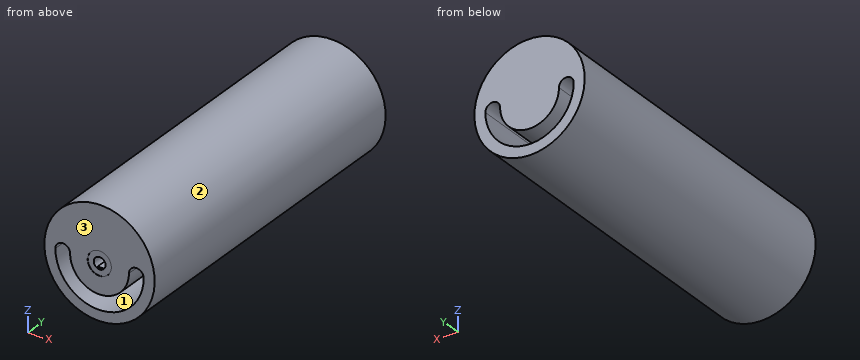
```python
from build123d import *

# Parameters (mm, degrees)
SKETCH1_R           = 28.1
BOSS_EXTRUDE2_DEPTH = 61.3
SKETCH3_R           = 18.6
CUT_EXTRUDE2_DEPTH  = 58.8
SKETCH4_W           = 56.2
SKETCH4_H           = 56.2
BOSS_EXTRUDE3_DEPTH = 56.2
SKETCH5_R           = 16.1
CUT_EXTRUDE4_DEPTH  = 5
SKETCH6_W           = 49.797391422
SKETCH6_H           = 49.779255452
CUT_EXTRUDE5_DEPTH  = 53.7
SKETCH7_R           = 28.1
BOSS_EXTRUDE4_DEPTH = 321.5
CUT_EXTRUDE6_DEPTH  = 10
SKETCH9_R           = 3
CUT_EXTRUDE7_DEPTH  = 1
SKETCH10_R          = 6.025
CUT_EXTRUDE8_DEPTH  = 0.1
SKETCH18_R          = 3.75
CUT_EXTRUDE9_DEPTH  = 100
SKETCH19_R          = 3.75
CUT_EXTRUDE11_DEPTH = 325
SKETCH20_W          = 56.2
SKETCH20_H          = 56.2
CUT_EXTRUDE13_DEPTH = 200
SKETCH21_R          = 28.1
CUT_EXTRUDE14_DEPTH = 150


with BuildPart() as part:
    # Sketch1 → Boss-Extrude2 (new body)
    with BuildSketch(Plane.XY):
        Circle(SKETCH1_R)
    extrude(amount=BOSS_EXTRUDE2_DEPTH)

    # Sketch3 → Cut-Extrude2 (cut)
    with BuildSketch(Plane.XY.offset(61.3)):
        with Locations((0, -7)):
            Circle(SKETCH3_R)
    extrude(amount=-CUT_EXTRUDE2_DEPTH, mode=Mode.SUBTRACT)

    # Sketch4 → Boss-Extrude3 (add)
    with BuildSketch(Plane(origin=(0, 0, 0), x_dir=(-1, 0, 0), z_dir=(0, 0, -1))):
        Rectangle(SKETCH4_W, SKETCH4_H)
    extrude(amount=BOSS_EXTRUDE3_DEPTH)

    # Sketch5 → Cut-Extrude4 (cut)
    with BuildSketch(Plane.XY.offset(2.5)):
        with Locations((0, -7)):
            Circle(SKETCH5_R)
    extrude(amount=-CUT_EXTRUDE4_DEPTH, mode=Mode.SUBTRACT)

    # Sketch6 → Cut-Extrude5 (cut)
    with BuildSketch(Plane(origin=(0, 0, -56.2), x_dir=(-1, 0, 0), z_dir=(0, 0, -1))):
        Rectangle(SKETCH6_W, SKETCH6_H)
    extrude(amount=-CUT_EXTRUDE5_DEPTH, mode=Mode.SUBTRACT)

    # Sketch7 → Boss-Extrude4 (add)
    with BuildSketch(Plane(origin=(0, -28.1, 0), x_dir=(-1, 0, 0), z_dir=(0, -1, 0))):
        with Locations(Location((0, 28.1, 0), (0, 0, 90))):
            Circle(SKETCH7_R)
    extrude(amount=BOSS_EXTRUDE4_DEPTH)

    # Sketch8 → Cut-Extrude6 (cut)
    with BuildSketch(Plane(origin=(0, -349.6, 0), x_dir=(-1, 0, 0), z_dir=(0, -1, 0))):
        with BuildLine():
            Line((-1.658312395, 25.832078896), (1.658312395, 25.832078896))
            ThreePointArc((1.658312395, 25.832078896), (3, 28.332078896), (1.658312395, 30.832078896))
            Line((1.658312395, 30.832078896), (-1.658312395, 30.832078896))
            ThreePointArc((-1.658312395, 30.832078896), (-3, 28.332078896), (-1.658312395, 25.832078896))
        make_face()
    extrude(amount=-CUT_EXTRUDE6_DEPTH, mode=Mode.SUBTRACT)

    # Sketch9 → Cut-Extrude7 (cut)
    with BuildSketch(Plane(origin=(0, -349.6, 0), x_dir=(-1, 0, 0), z_dir=(0, -1, 0))):
        with Locations(Location((0, 28.332078896, 0), (0, 0, 90))):
            Circle(SKETCH9_R)
    extrude(amount=-CUT_EXTRUDE7_DEPTH, mode=Mode.SUBTRACT)

    # Sketch10 → Cut-Extrude8 (cut)
    with BuildSketch(Plane(origin=(0, -349.6, 0), x_dir=(-1, 0, 0), z_dir=(0, -1, 0))):
        with Locations(Location((0, 28.332078896, 0), (0, 0, 90))):
            Circle(SKETCH10_R)
    extrude(amount=-CUT_EXTRUDE8_DEPTH, mode=Mode.SUBTRACT)

    # Cut-Sweep4: sweep along a path in Sketch15
    with BuildLine(Plane(origin=(0, -349.6, 0), x_dir=(-1, 0, 0), z_dir=(0, -1, 0))) as cut_sweep4_path:
        ThreePointArc((15, 28.332078896), (0, 43.332078896), (-15, 28.332078896))
    # 3DSketch2 → Cut-Sweep4 (sweep, cut)
    with BuildSketch(Plane(origin=(-15, -349.6, -28.332078896), x_dir=(-0.022748965612757834, 0.999741208795331, 0), z_dir=(0, 0, 1))):
        Polygon((0, 0), (0.170617242, 7.498059066), (329.685319661, 0), (329.514702419, -7.498059066), align=None)
    sweep(path=cut_sweep4_path.line, mode=Mode.SUBTRACT)

    # Sketch18 → Cut-Extrude9 (cut)
    with BuildSketch(Plane.XY.offset(61.3)):
        with Locations((0, 18.75)):
            Circle(SKETCH18_R)
    extrude(amount=-CUT_EXTRUDE9_DEPTH, mode=Mode.SUBTRACT)

    # Sketch19 → Cut-Extrude11 (cut)
    with BuildSketch(Plane(origin=(0, -349.6, 0), x_dir=(-1, 0, 0), z_dir=(0, -1, 0))):
        with Locations((-18.75, 28.332078896)):
            Circle(SKETCH19_R)
        with Locations((18.75, 28.332078896)):
            Circle(SKETCH19_R)
    extrude(amount=-CUT_EXTRUDE11_DEPTH, mode=Mode.SUBTRACT)

    # Sketch20 → Cut-Extrude13 (cut)
    with BuildSketch(Plane(origin=(0, 0, -56.2), x_dir=(-1, 0, 0), z_dir=(0, 0, -1))):
        Rectangle(SKETCH20_W, SKETCH20_H)
    extrude(amount=-CUT_EXTRUDE13_DEPTH, mode=Mode.SUBTRACT)

    # Sketch21 → Cut-Extrude14 (cut)
    with BuildSketch(Plane(origin=(0, -28.1, 0), x_dir=(1, 0, 0), z_dir=(0, 1, 0))):
        with Locations(Location((0, 28.1, 0), (0, 0, 270))):
            Circle(SKETCH21_R)
    extrude(amount=-CUT_EXTRUDE14_DEPTH, mode=Mode.SUBTRACT)


solid = part.part
```
The listing builds one solid part. Answer for the finished solid, in the listing's coordinates (mm). Face numbers are marked on the shaded views. Give positions to 0.01 mm unless a question says otherwise; leave off trailing zeros. Write each loop counter-clockwise with the first axis right and the second up, starting at its lowest first coordinate (ties: lowest second). Pieces come first, ordered by that corner, then holes. Notation, with made-up numbers: (14.25, 27) -> (35.25, 27) arc R26 ccw to (35.25, 64) -> close; hole circle Ø5 at (76.5, 84). An arc over 180 degrees is marked (long way). Use one line per item in the form item = value.
1) Section D-D on z = -16 is taken. Write down the section's boundary in (x, y).
Result:
outline = (-25.36, -349.6) -> (25.36, -349.6) -> (25.36, -178.1) -> (-25.36, -178.1) -> close
2) Section B-B on y = -238 is taken. Write down the section's boundary in (x, z), plus the area to 3 significant figures.
Result:
outline = circle Ø56.2 at (0, -28.1); hole (-22.5, -28.33) arc R22.5 ccw to (22.5, -28.33) arc R3.75 ccw to (15, -28.33) arc R15 cw to (-15, -28.33) arc R3.75 ccw to start
area = 1,990 mm²
3) Section A-A on x = 0 is taken. Write down the section's boundary in (y, z), plus the area to 3 significant figures.
Result:
outline = (-349.6, -56.2) -> (-178.1, -56.2) -> (-178.1, -50.83) -> (-349.6, -50.83) -> close; (-349.6, -43.33) -> (-178.1, -43.33) -> (-178.1, 0) -> (-349.6, 0) -> (-349.6, -22.31) -> (-349.5, -22.31) -> (-349.5, -25.33) -> (-348.6, -25.33) -> (-348.6, -25.83) -> (-339.6, -25.83) -> (-339.6, -30.83) -> (-348.6, -30.83) -> (-348.6, -31.33) -> (-349.5, -31.33) -> (-349.5, -34.36) -> (-349.6, -34.36) -> close
area = 8,300 mm²
4) For a pull along X with two mould halves and no side action, classify the marked faces 1, 2 and 3 as +X half, -X half, draft (parallel to the pull), parting line (faces both ways), or undercut.
Result:
face_1 = undercut
face_2 = parting line
face_3 = draft
5) Section C-C on x = -20 is taken. Write down the section's boundary in (y, z), plus the area to 3 significant figures.
Result:
outline = (-349.6, -47.84) -> (-178.1, -47.84) -> (-178.1, -38.64) -> (-349.6, -38.64) -> close; (-349.6, -24.8) -> (-178.1, -24.8) -> (-178.1, -8.36) -> (-349.6, -8.36) -> close
area = 4,400 mm²
6) Straight lines are drawn through the part: probe 1 along X at (y, z) = (-324.5, -29); probe 2 along X at (y, z) = (-298.5, -33.5); probe 3 along Y at (x, z) = (0.5, -34). For each, find the intervals that lie inside material, in ascending order.
Result:
probe_1 = -28.09 to -22.49, -14.99 to 14.99, 22.49 to 28.09
probe_2 = -27.58 to -21.9, -14.08 to 14.08, 21.9 to 27.58
probe_3 = -349.5 to -178.1
7) Each of these flat-tipped pins is pushed along its axis until it touches: P1, Ø12, axis at y = -283, z = -45, coming from the -X side; P2, Ø3, axis at y = -237.5, z = -43, coming from the -X side; P3, Ø8, axis at x = 13.5, y = -310, coming from the -Z side. Where does it stop, or does it pass through?
Result:
P1 = -25.9
P2 = -24.7
P3 = -54.55
